Autodesk Inventor part; units mm, degrees
ref_plane "mirror door slot" through (-254, 25.4, 0) normal (1, 0, 0) x (0, 0, -1)
ref_plane "YZ Plane" through (0, 0, 0) normal (1, 0, 0) x (0, 1, 0)
ref_plane "XZ Plane" through (0, 0, 0) normal (0, 1, 0) x (-1, 0, 0)
sketch "Sketch1" plane through (0, 0, 0) normal (0, 1, 0) x (-1, 0, 0)
  line L0 (0, 0) -> (508, 0)
  line L1 (508, 0) -> (508, -635)
  line L2 (508, -635) -> (0, -635)
  line L3 (0, -635) -> (0, 0)
  dimension "d0" = 508
  dimension "d1" = 635
extrude "floor" add sketch "Sketch1" along normal blind 25.4
sketch "Sketch4" plane through (0, 25.4, 0) normal (0, 1, 0) x (1, 0, 0)
  line L0 (-508, 0) -> (0, 0)
  line L1 (0, 0) -> (0, 635)
  line L2 (0, 0) -> (0, 635)
  line L3 (0, 635) -> (-508, 635)
  line L4 (0, 635) -> (-508, 635)
  line L5 (-508, 635) -> (-508, 0)
  line L6 (-508, 0) -> (0, 0)
  line L7 (-25.4, 25.4) -> (-482.6, 25.4)
  line L8 (-482.6, 25.4) -> (-482.6, 609.6)
  line L9 (-482.6, 609.6) -> (-25.4, 609.6)
  line L10 (-25.4, 609.6) -> (-25.4, 25.4)
  dimension "d11" = 25.4
  dimension "d12" = 25.4
  dimension "d13" = 25.4
  dimension "d14" = 25.4
extrude "walls" add sketch "Sketch4" along normal blind 220.1333
sketch "Sketch5" plane through (-508, 0, 0) normal (0, 0, 1) x (1, 0, 0)
  line L0 (25.4, 25.4) -> (482.6, 25.4)
  line L1 (254, 25.4) -> (304.8, 25.4)
  line L2 (304.8, 25.4) -> (304.8, 194.7333)
  line L3 (304.8, 194.7333) -> (254, 194.7333)
  line L4 (254, 194.7333) -> (254, 25.4)
  line L5 (254, 25.4) -> (203.2, 25.4)
  line L6 (203.2, 25.4) -> (203.2, 194.7333)
  line L7 (203.2, 194.7333) -> (254, 194.7333)
  point P0 (508, 0)
  dimension "d17" = 50.8
  dimension "d18" = 169.3333
extrude "doorframe" cut sketch "Sketch5" against normal blind 220.1333
sketch "Sketch7" plane through (0, 245.5333, 0) normal (0, 1, 0) x (1, 0, 0)
  line L0 (-482.6, 25.4) -> (-482.6, 609.6)
  line L1 (-25.4, 25.4) -> (-25.4, 609.6)
  line L2 (-482.6, 609.6) -> (-25.4, 609.6)
  line L3 (-25.4, 609.6) -> (-25.4, 25.4)
  line L4 (-25.4, 25.4) -> (-482.6, 25.4)
  line L5 (-482.6, 25.4) -> (-482.6, 609.6)
  point P0 (0, 0)
extrude "ceiling" add sketch "Sketch7" against normal blind 25.4
sketch "Sketch8" plane through (-304.8, 25.4, 0) normal (1, 0, 0) x (0, 0, -1)
  line L0 (12.7, 169.3333) -> (19.05, 169.3333)
  line L1 (19.05, 169.3333) -> (19.05, 0)
  line L2 (19.05, 0) -> (6.35, 0)
  line L3 (6.35, 0) -> (6.35, 169.3333)
  line L4 (12.7, 169.3333) -> (6.35, 169.3333)
  point P0 (0, -25.4)
  point P1 (0, 169.3333)
  point P2 (25.4, 169.3333)
  point P3 (0, 0)
  point P4 (25.4, 0)
  dimension "d24" = 6.35
  dimension "d25" = 12.7
  dimension "d28" = 169.3333
extrude "left door slot" cut sketch "Sketch8" against normal blind 50.8
ref_plane "mirror door slot" through (-254, 25.4, 0) normal (1, 0, 0) x (0, 0, -1)
mirror "right door slot" about plane through (-254, 25.4, 0) normal (1, 0, 0) of "left door slot"
sketch "Sketch10" plane through (-508, 0, 0) normal (0, 0, 1) x (1, 0, 0)
  line L0 (203.2, 194.7333) -> (304.8, 194.7333)
  line L1 (203.2, 25.4) -> (304.8, 25.4)
  arc A0 (311.4059, 0) -> (196.5941, 0) centre (254, 110.0667) ccw
  arc A1 (203.2, 194.7333) -> (203.2, 25.4) centre (254, 110.0667) ccw
  arc A2 (304.8, 25.4) -> (304.8, 194.7333) centre (254, 110.0667) ccw
  line L2 (203.2, 194.7333) -> (304.8, 194.7333)
  line L3 (203.2, 194.7333) -> (203.2, 25.4)
  line L4 (508, 0) -> (0, 0)
  line L5 (196.5941, 0) -> (311.4059, 0)
  point P0 (254, 194.7333)
  point P1 (203.2, 110.0667)
  dimension "d37" = 169.3333
  dimension "d38" = 101.6
  dimension "d39" = 25.4
extrude "corridor connect" add sketch "Sketch10" along normal blind 25.4
equation "\"d12\" = d11"
equation "\"d13\" = d12"
equation "\"d14\" = d13"
properties part number "main room"
CAD build for the part. Positions are in the model's coordinates, mm. A direction names the side the tool comes from. Give positions to 0.01 mm unless a question says otherwise; leave off trailing zeros. Write each loop counter-clockwise with the first axis right and the second up, starting at its lowest first coordinate (ties: lowest second). Pieces come first, ordered by that corner, then holes. Notation, with made-up numbers: M -36,32 L -10,32 A13 ccw -10,47 Z; hole C 44.5,43 d5. An arc over 180 degrees is marked long. Return JSON: item names as keys, results as strings. Group by question number.
(1) Band-saw the part on B-B (x = -475.5). Give the cut face in (y, z).
(2) 3-axis set-ups, long thin cutter, end or side, ignore diameter. For faces 1 (the face through (-25.4, 121, -322)), 2 (the face through (-323, 109, 0)), 3 (the face through (-508, 121, -313)): which of +Z, -Z, +X, -X, +Y, -Y reach the whole face in a straight line?
(3) Band-saw the part on D-D (y = 163). Give the cut face in (x, z).
(4) Mould opens along Y. For faces 4 (the face through (0, 121, -322)), 5 (the face through (-250, 0, -309)), 6 (the face through (-257, 25.4, -297)), 7 (the face through (-155.273, 111.491, 12.522)) say: pulls with the +Y half, pulls with the -Y half, needs draft (parallel to the pull), parting line crosses it, or undercut.
(5) Band-saw the part on C-C (x = -254). Give the cut face in (y, z), and give its area (3 significant figures).
(6) Drill centre lines: L1, parallel to Y at x = -106.5, z = -516; L2, parallel to X at y = 114, z = -93; L3, parallel to Z at x = -479.5, y = 81. Where is each one in solid material? Low to high. Write a range as [from, to].
(7) Flat gauge pins, fed straight in: pin 1 Ø3 at (x, z) = (-301, -551.5) entering from -Y; pin 2 Ø6 at (x, y) = (-321, 138.5) entering from +Z. Where does each tip first touch, or does it go through?
(8) Band-saw the part on A-A (z = -283). Give the cut face in (x, y), and give its area (3 significant figures).
Entries:
{
 "1": {"outline": "M 0,-635 L 245.53,-635 L 245.53,0 L 0,0 Z; hole M 25.4,-609.6 L 220.13,-609.6 L 220.13,-25.4 L 25.4,-25.4 Z"},
 "2": {"face 1": "none", "face 2": "+Z", "face 3": "+Z, -Z, -X, +Y, -Y"},
 "3": {"outline": "M -508,-635 L 0,-635 L 0,0 L -141.71,0 L -141.71,25.4 L -170.65,25.4 L -170.65,0 L -203.2,0 L -203.2,-6.35 L -152.4,-6.35 L -152.4,-19.05 L -203.2,-19.05 L -203.2,-25.4 L -25.4,-25.4 L -25.4,-609.6 L -482.6,-609.6 L -482.6,-25.4 L -304.8,-25.4 L -304.8,-19.05 L -355.6,-19.05 L -355.6,-6.35 L -304.8,-6.35 L -304.8,0 L -337.35,0 L -337.35,25.4 L -366.29,25.4 L -366.29,0 L -508,0 Z"},
 "4": {"face 4": "needs draft", "face 5": "pulls with the -Y half", "face 6": "undercut", "face 7": "undercut"},
 "5": {"outline": "M 0,-635 L 245.53,-635 L 245.53,0 L 234.2,0 L 234.2,25.4 L 194.73,25.4 L 194.73,-25.4 L 220.13,-25.4 L 220.13,-609.6 L 25.4,-609.6 L 25.4,25.4 L 0,25.4 Z", "area": "39,500 mm^2"},
 "6": {"L1": "y = [0, 25.4], [220.13, 245.53]", "L2": "x = [-508, -482.6], [-25.4, 0]", "L3": "z = [-635, -609.6], [-25.4, 0]"},
 "7": {"pin 1": "stops at y = 0", "pin 2": "stops at z = 0"},
 "8": {"outline": "M -508,0 L 0,0 L 0,245.53 L -508,245.53 Z; hole M -482.6,25.4 L -25.4,25.4 L -25.4,220.13 L -482.6,220.13 Z", "area": "35,700 mm^2"}
}
